Model file for the job. Use its own axes, mm. A direction names the side the tool comes from. Coordinates: 2 decimals unless noted, no trailing zeros. Order: outer loops, then holes, each group sorted by start corner. A loop starts at its lowest first (then second) coordinate and runs counter-clockwise, first axis right, second up. Notation, with made-up numbers: (-9, 12) -> (17, 12) arc R22 cw to (17, 46) -> close; hole circle Ø10 at (-10.5, 54.25). An arc over 180 degrees is marked (long way). Return JSON: item names as keys, results as strings. Group by question number.
1) Cut at C-C (y = -22.5). Write the cut outline in (x, z).
2) Which spindle directions (+Z, -Z, +X, -X, +Y, -Y) get a long thin tool onto all of the face, cutting with end or side? Do faces 1 (the cylindrical face through (-12.367, -32.136, 6.45)), 2 (the flat face through (1, -28, 13.12)). Say none if no direction does.
3) Cut at D-D (z = 1.5). Write the cut outline in (x, y), and give its area (3 significant figures).
4) Cut at A-A (x = 3.5). Write the cut outline in (y, z), and give its area (3 significant figures).
5) Pull direction Z, two halves, no side cores. Call faces 3 (the conical face through (-9.52, -23.76, 6.82)), 4 (the cylindrical face through (-17.719, -20.28, 2.406)), 5 (the cylindrical face through (-19.14, -25.05, 12.22)): +Z half, -Z half, draft (parallel to the pull), parting line (faces both ways), or undercut.
6) Probe line 1 (Z direction, x = 13, y = -28); line 2 (X direction, y = -34.5, z = 4.5); line 3 (Z direction, x = 15, y = -28.5). List the from-to ranges inside material, lowest first.
7) Cut at B-B (y = -31.5). Write the cut outline in (x, z).
8) Flat gauge pin, fed straight in: pin 1 (4 mm diameter, centred on y = -34, z = 2, fed in from -X). Where does the tip first touch, or does it go through?
from build123d import *

# Parameters (mm, degrees)
BOSS_EXTRUDE1_DEPTH         = 20
FILLET1_R                   = 1
FILLET2_R                   = 2
FILLET3_R                   = 8
FILLET4_R                   = 3
M6_TAPPED_HOLE1_D           = 5
M6_TAPPED_HOLE1_DEPTH       = 15
M6_TAPPED_HOLE1_CSINK_D     = 6.05
M6_TAPPED_HOLE1_CSINK_ANGLE = 90
M6_TAPPED_HOLE1_TIP         = 1.502151548


with BuildPart() as part:
    # Sketch1 → Boss-Extrude1 (new, symmetric)
    with BuildSketch(Plane(origin=(0, 0, 0), x_dir=(0, 0, -1), z_dir=(1, 0, 0))):
        with BuildLine():
            Line((-5, 0), (0, 0))
            Line((0, 0), (0, -40))
            Line((0, -40), (-13.12, -40))
            Line((-13.12, -40), (-13.12, -15))
            Line((-13.12, -15), (-11.32121885, -15))
            Line((-11.32121885, -15), (-7.897777479, -2.223542865))
            ThreePointArc((-7.897777479, -2.223542865), (-6.826284287, -0.619939979), (-5, 0))
        make_face()
    extrude(amount=BOSS_EXTRUDE1_DEPTH, both=True)

    # Fillet1
    fillet1_edges = [part.edges().sort_by_distance(p)[0] for p in [
        (20, -27.5, 13.12),
        (20, -20, 0),
    ]]
    fillet(fillet1_edges, radius=FILLET1_R)

    # Fillet2
    fillet2_edges = [part.edges().sort_by_distance(p)[0] for p in [
        (0, -15, 11.32121885),
    ]]
    fillet(fillet2_edges, radius=FILLET2_R)

    # Fillet3
    fillet3_edges = [part.edges().sort_by_distance(p)[0] for p in [
        (-20, -20, 0),
    ]]
    fillet(fillet3_edges, radius=FILLET3_R)

    # Fillet4
    fillet4_edges = [part.edges().sort_by_distance(p)[0] for p in [
        (-20, -27.5, 13.12),
    ]]
    fillet(fillet4_edges, radius=FILLET4_R)

    # M6 Tapped Hole1
    with Locations(Plane(origin=(0, -40, 0), x_dir=(-1, 0, 0), z_dir=(0, -1, 0))):
        with Locations((-13, -6.56), (9.869332882, -6.56)):
            CounterSinkHole(M6_TAPPED_HOLE1_D / 2, M6_TAPPED_HOLE1_CSINK_D / 2, depth=M6_TAPPED_HOLE1_DEPTH, counter_sink_angle=M6_TAPPED_HOLE1_CSINK_ANGLE)
            with Locations((0, 0, -(M6_TAPPED_HOLE1_DEPTH + M6_TAPPED_HOLE1_TIP / 2))):  # 118° drill point
                Cone(0, M6_TAPPED_HOLE1_D / 2, M6_TAPPED_HOLE1_TIP, mode=Mode.SUBTRACT)


solid = part.part
Answers below:
{
 "1": {"outline": "(-20, 8) arc R8 ccw to (-12, 0) -> (19, 0) arc R1 ccw to (20, 1) -> (20, 12.12) arc R1 ccw to (19, 13.12) -> (-17, 13.12) arc R3 ccw to (-20, 10.12) -> close"},
 "2": {"face 1": "-Y", "face 2": "+Z, +X, -X, +Y, -Y"},
 "3": {"outline": "(-16.66, -40) -> (20, -40) -> (20, 0) -> (-16.66, 0) -> close", "area": "1,470 mm^2"},
 "4": {"outline": "(-40, 0) -> (0, 0) -> (0, 5) arc R3 ccw to (-2.22, 7.9) -> (-13.52, 10.92) arc R2 cw to (-15, 12.86) -> (-15, 13.12) -> (-40, 13.12) -> close", "area": "467 mm^2"},
 "5": {"face 3": "undercut", "face 4": "-Z half", "face 5": "+Z half"},
 "6": {"line 1": "z = 0 to 4.06, 9.06 to 13.12", "line 2": "x = -19.19 to -11.29, -8.45 to 11.58, 14.42 to 20", "line 3": "z = 0 to 5.06, 8.06 to 13.12"},
 "7": {"outline": "(-20, 8) arc R8 ccw to (-12, 0) -> (19, 0) arc R1 ccw to (20, 1) -> (20, 12.12) arc R1 ccw to (19, 13.12) -> (-17, 13.12) arc R3 ccw to (-20, 10.12) -> close; hole circle Ø5 at (-9.87, 6.56); hole circle Ø5 at (13, 6.56)"},
 "8": {"pin 1": "stops at x = -18.93"}
}
